from build123d import *

# Parameters (mm, degrees)
CUT_EXTRUDE1_DEPTH = 3


with BuildPart() as part:
    # Sketch1 → Revolve1 (revolve)
    with BuildSketch(Plane.XY, mode=Mode.PRIVATE) as revolve1_sk:
        Polygon((0, 0), (-22.225, 0), (-22.225, 2.1082), (0, 63.170885647), (0, 60.127205267), (-20.064661815, 5), (0, 5), align=None)
    revolve(revolve1_sk.sketch.rotate(Axis((0, 0, 0), (0, 1, 0)), 270), axis=Axis((0, 0, 0), (0, 1, 0)))

    # Sketch9 → Revolve3 (revolve)
    with BuildSketch(Plane.XY, mode=Mode.PRIVATE) as revolve3_sk:
        Polygon((-22.1611, 0), (-22.1611, -15), (-21.1201, -15), (-21.1201, 2.1082), (-23.2021, 2.1082), (-23.2021, 0), align=None)
    revolve(revolve3_sk.sketch.rotate(Axis((0, 63.536813388, 0), (0, -1, 0)), 270), axis=Axis((0, 63.536813388, 0), (0, -1, 0)))

    # Sketch10 → Cut-Extrude1 (cut)
    with BuildSketch(Plane.XZ):
        Polygon((-5.25, 13.25), (5.25, 13.25), (5.25, 10.25), (16.25, 10.25), (16.25, -10.25), (5.25, -10.25), (5.25, -13.25), (-5.25, -13.25), (-5.25, -10.25), (-16.25, -10.25), (-16.25, 10.25), (-5.25, 10.25), align=None)
    extrude(amount=-CUT_EXTRUDE1_DEPTH, mode=Mode.SUBTRACT)


solid = part.part
Input: part model. Units: mm. Frame: model coordinates. A direction names the side the tool comes from. Coordinates: 2 decimals unless noted, no trailing zeros. Loops run counter-clockwise (first coordinate to the right, second up) from the corner with the lowest first, then second, coordinate; pieces in that order, holes last. Notation, with made-up numbers: (87, 1.25) - (111, 1.25) arc R25 cw to (111, 40.25) - close; hole circle Ø11 at (-1.75, 64). An arc over 180 degrees is marked (long way). Answer in a Markdown table with one row per item. Add a question column.
Item 1: Line query: line 1 along X through (y, z) = (-7, 0); line 2 along Y through (x, z) = (4, -8.5); line 3 along Y through (x, z) = (-11.5, 15.5). Output: solid intervals per line, ascending. Write a range as [from, to].
Item 2: Access query for faces 4 (the flat face through (5.25, 1, 12)), 5 (the conical face through (7.754, 38.303, 1.722)), 6 (the cylindrical face through (22.65, 1.04, -5.03)). Directions: +Z, -Z, +X, -X, +Y, -Y. A direction counts if a zero-diameter tool reaches every point of the face in a straight line with its end or side. Return the directions, or none.
Item 3: Contact query for flat-ended pins moving along their axis: P1, Ø8, axis at x = 14.5, z = 8.5, coming from the -Y side; P2, Ø10, axis at x = -10, y = 4, coming from the -Z side; P3, Ø8, axis at x = 12, y = 5, coming from the +Z side; P4, Ø23, axis at x = -2.5, z = -10, coming from the -Y side. Output: stop coordinate, or through.
Item 4: Section query A-A on y = -5. Return the cut outline in (x, z), then the cut area to 3 significant figures.
Item 5: Mould query, pull axis Y, two halves, no side actions, for faces 1 (the flat face through (0, 5, 0)), 2 (the flat face through (-16.25, 1, 0)), 3 (the flat face through (19, 2.108, -12)). Classes: released by +Y, released by -Y, zero draft, split by the parting line, or undercut.
Item 6: Section query B-B on y = 56.5. Return the cut outline in (x, z), then the cut area to 3 significant figures.
Recorded:
| question | item | result |
|---|---|---|
| 1 | line 1 | [-22.16, -21.12], [21.12, 22.16] |
| 1 | line 2 | [3, 5], [34.32, 37.36] |
| 1 | line 3 | [0, 5], [7.1, 10.14] |
| 2 | face 4 | -Y |
| 2 | face 5 | none |
| 2 | face 6 | +Y, -Y |
| 3 | P1 | y = 0 |
| 3 | P2 | z = -22.57 |
| 3 | P3 | z = 21.28 |
| 3 | P4 | y = -15 |
| 4 | outline | circle Ø44.32 at (0, 0); hole circle Ø42.24 at (0, 0) |
| 4 | area | 142 mm^2 |
| 5 | face 1 | undercut |
| 5 | face 2 | zero draft |
| 5 | face 3 | released by +Y |
| 6 | outline | circle Ø4.86 at (0, 0); hole circle Ø2.64 at (0, 0) |
| 6 | area | 13.0 mm^2 |
